The model under review builds one solid part; all positions refer to its coordinate system, in mm. Face numbers are marked on the shaded views. A direction names the side the tool comes from. Round coordinates to 2 decimals unless told otherwise and drop trailing zeros. Write each loop counter-clockwise with the first axis right and the second up, starting at its lowest first coordinate (ties: lowest second). Pieces come first, ordered by that corner, then holes. Notation, with made-up numbers: (2, 2.25) - (21, 2.25) arc R25 cw to (21, 31.25) - close; hole circle Ø1 at (-26, 40). An arc over 180 degrees is marked (long way). Return JSON: item names as keys, results as strings.
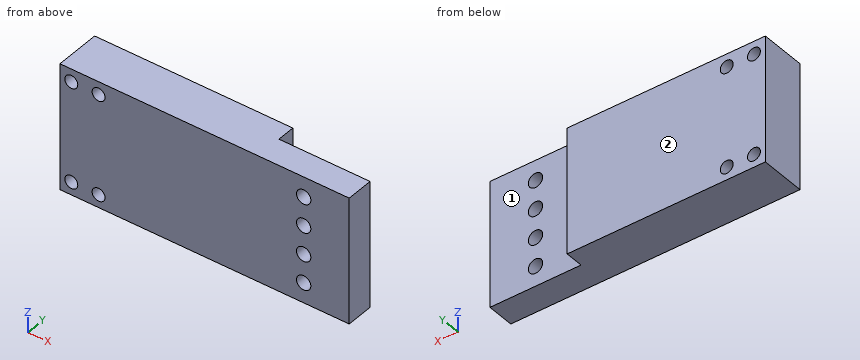
from build123d import *

# Parameters (mm, degrees)
F0_W     = 201.639
F0_H     = 88
F1_DEPTH = 31.75
F2_W     = 63.5
F2_H     = 12.7
F3_DEPTH = 88.001
F4_R     = 4.5
F4_R_2   = 5
F5_DEPTH = 31.751


with BuildPart() as f1:
    # F0 (on Front) → F1 (new body)
    with BuildSketch(Plane.XZ):
        with Locations((-3.479119, -15.731822)):
            Rectangle(F0_W, F0_H)
    extrude(amount=F1_DEPTH)

    # F2 (on face) → F3 (cut, through all)
    with BuildSketch(Plane(origin=(0, 0, -59.731822), x_dir=(1, 0, 0), z_dir=(0, 0, -1))):
        with Locations((65.590381, 6.35)):
            Rectangle(F2_W, F2_H)
    extrude(amount=-F3_DEPTH, mode=Mode.SUBTRACT)

    # F4 (on face) → F5 (cut, through all)
    with BuildSketch(Plane.XZ.offset(31.75)):
        with Locations((-96.376619, -50.731822)):
            Circle(F4_R)
        with Locations((-96.376619, 19.268178)):
            Circle(F4_R)
        with Locations((-77.376619, -50.731822)):
            Circle(F4_R)
        with Locations((-77.376619, 19.268178)):
            Circle(F4_R)
        with Locations((65.590381, -45.731822)):
            Circle(F4_R_2)
        with Locations((65.590381, -25.731822)):
            Circle(F4_R_2)
        with Locations((65.590381, -5.731822)):
            Circle(F4_R_2)
        with Locations((65.590381, 14.268178)):
            Circle(F4_R_2)
    extrude(amount=-F5_DEPTH, mode=Mode.SUBTRACT)


solid = f1.part
(1) For the marked faces 1 and 2, list the 3-axis set-ups (+Z, -Z, +X, -X, +Y, -Y) from which the entire face can be reached by the end or side of a thin tool; tool diameter is ignored.
Filled in:
{"face 1": "+Z, -Z, +X, +Y", "face 2": "+Z, -Z, +X, -X, +Y"}
(2) Wall thickness on line 1 (X direction, y = -16.5, z = -54); line 2 (Z direction, x = -78.5, y = -19); line 3 (Z direction, x = -95, y = -13): over which ranges is each line inside the solid? List them lowest first.
Filled in:
{"line 1": "x = -104.3 to -99.47, -93.28 to -80.47, -74.28 to 97.34", "line 2": "z = -59.73 to -55.09, -46.37 to 14.91, 23.63 to 28.27", "line 3": "z = -59.73 to -55.02, -46.45 to 14.98, 23.55 to 28.27"}
(3) Add section D-D (x = -78). Write out the cut boundary in (y, z), plus the area to 3 significant figures.
Filled in:
{"outline": "(-31.75, -59.73) - (0, -59.73) - (0, -55.19) - (-31.75, -55.19) - close; (-31.75, -46.28) - (0, -46.28) - (0, 14.81) - (-31.75, 14.81) - close; (-31.75, 23.72) - (0, 23.72) - (0, 28.27) - (-31.75, 28.27) - close", "area": "2,230 mm2"}
(4) Clearance check with flat-ended pins moving along their axes: pin 1 Ø6 at (x, z) = (-17, -5) entering from +Y; pin 2 Ø16 at (x, z) = (65.59, -5.73) entering from +Y; pin 3 Ø14 at (y, z) = (-4, 1) entering from +X; pin 4 Ø5.5 at (x, z) = (-96.38, 19.27) entering from +Y. State where each tip first meets the part, or that it passes through.
Filled in:
{"pin 1": "stops at y = 0", "pin 2": "stops at y = -12.7", "pin 3": "stops at x = 33.84", "pin 4": "passes through"}
(5) Add section A-A (y = -10). Write out the cut boundary in (x, z).
Filled in:
{"outline": "(-104.3, -59.73) - (33.84, -59.73) - (33.84, 28.27) - (-104.3, 28.27) - close; hole circle Ø9 at (-96.38, -50.73); hole circle Ø9 at (-96.38, 19.27); hole circle Ø9 at (-77.38, -50.73); hole circle Ø9 at (-77.38, 19.27)"}
(6) Add section B-B (z = -53). Write out the cut boundary in (x, y).
Filled in:
{"outline": "(-104.3, -31.75) - (-100.26, -31.75) - (-100.26, 0) - (-104.3, 0) - close; (-92.49, -31.75) - (-81.26, -31.75) - (-81.26, 0) - (-92.49, 0) - close; (-73.49, -31.75) - (97.34, -31.75) - (97.34, -12.7) - (33.84, -12.7) - (33.84, 0) - (-73.49, 0) - close"}
(7) Add section C-C (z = -43). Write out the cut boundary in (x, y), plus the area to 3 significant figures.
Filled in:
{"outline": "(-104.3, -31.75) - (61.4, -31.75) - (61.4, -12.7) - (33.84, -12.7) - (33.84, 0) - (-104.3, 0) - close; (69.78, -31.75) - (97.34, -31.75) - (97.34, -12.7) - (69.78, -12.7) - close", "area": "5,440 mm2"}
